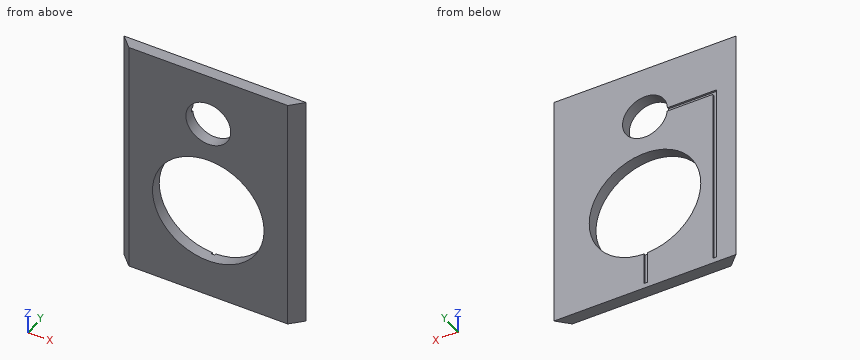
```python
from build123d import *

# Parameters (mm, degrees)
F0_W     = 300
F0_H     = 400
F1_DEPTH = 19
F2_R     = 37
F2_R_2   = 92
F3_DEPTH = 19
F4_SIZE  = 18.99999
F6_DEPTH = 3
F7_W     = 6
F7_H     = 64.6666483516
F8_DEPTH = 3


# Not quite as in the source:
# - a fillet or chamfer is up to 0.001 mm smaller than in the source, because OpenCascade refuses the exact size


with BuildPart() as f1:
    # F0 (on Front) → F1 (new body)
    with BuildSketch(Plane.XZ):
        with Locations((-100.0432893634, -3.2491389651)):
            Rectangle(F0_W, F0_H)
    extrude(amount=F1_DEPTH)

    # F2 (on face) → F3 (cut)
    with BuildSketch(Plane.XZ.offset(19)):
        with Locations((-100.0432893634, 109.7508610349)):
            Circle(F2_R)
        with Locations((-100.0432893634, -48.7491389651)):
            Circle(F2_R_2)
    extrude(amount=-F3_DEPTH, mode=Mode.SUBTRACT)

    # F4 (size 19 in the source; OpenCascade refuses exactly that, so slightly less here)
    f4_edges = [f1.edges().sort_by_distance(p)[0] for p in [
        (-250.043289, -19, -3.249139),
        (49.956711, -19, -3.249139),
    ]]
    chamfer(f4_edges, length=F4_SIZE)

    # F5 (on face) → F6 (cut)
    with BuildSketch(Plane(origin=(0, 0, 0), x_dir=(-1, 0, 0), z_dir=(0, 1, 0))):
        Polygon((136.7686212203, 111.2508610349), (136.7686212203, 105.2508610349), (212.0432893634, 105.2508610349), (212.0432893634, -194.7491389651), (218.0432893634, -194.7491389651), (218.0432893634, 111.2508610349), align=None)
    extrude(amount=-F6_DEPTH, mode=Mode.SUBTRACT)

    # F7 (on face) → F8 (cut)
    with BuildSketch(Plane(origin=(0, 0, 0), x_dir=(-1, 0, 0), z_dir=(0, 1, 0))):
        with Locations((101.5432893634, -162.4158147893)):
            Rectangle(F7_W, F7_H)
    extrude(amount=-F8_DEPTH, mode=Mode.SUBTRACT)


solid = f1.part
```
Input: part model. Units: mm. Frame: model coordinates. Coordinates: 2 decimals unless noted, no trailing zeros. Order: outer loops, then holes, each group sorted by start corner. A loop starts at its lowest first (then second) coordinate and runs counter-clockwise, first axis right, second up. Notation, with made-up numbers: (-24.75, -7) - (-11.75, -7) arc R28 cw to (-11.75, 16) - close; hole circle Ø2 at (-31, -32). An arc over 180 degrees is marked (long way). Put each result on its own line as item: value.
1. Cut plane B-B on x = -89.5. Return the cut outline in (y, z), then the cut area to 3 significant figures.
Report:
outline: (-19, -203.25) - (0, -203.25) - (0, -140.14) - (-19, -140.14) - close; (-19, 42.64) - (0, 42.64) - (0, 74.28) - (-19, 74.28) - close; (-19, 145.22) - (0, 145.22) - (0, 196.75) - (-19, 196.75) - close
area: 2,780 mm2
2. Cut plane D-D on y = -6.75. Return the cut outline in (x, z), then the cut area to 3 significant figures.
Report:
outline: (-243.29, -203.25) - (43.21, -203.25) - (43.21, 196.75) - (-243.29, 196.75) - close; hole circle Ø184 at (-100.04, -48.75); hole circle Ø74 at (-100.04, 109.75)
area: 83,700 mm2
3. Line query: line 1 along Z through (x, y) = (-90, -3.75); line 2 along Z through (x, y) = (-68, -9); line 3 along X through (y, z) = (-5.75, 143.5). Output: solid intervals per line, ascending.
Report:
line 1: z = -203.25 to -140.2, 42.7 to 74.14, 145.36 to 196.75
line 2: z = -203.25 to -134.99, 37.49 to 91.25, 128.25 to 196.75
line 3: x = -244.29 to -115.21, -84.88 to 44.21
4. Contact query for flat-ended pins moving along their axis: pin 1 Ø24.5 at (x, z) = (-174, -111.5) entering from +Y; pin 2 Ø3.5 at (y, z) = (-2, -159) entering from +X; pin 3 Ø2 at (y, z) = (-13.5, 103) entering from +X; pin 4 Ø1.8 at (x, z) = (-102.5, -179.5) entering from +Y. Output: stop coordinate, or through.
Report:
pin 1: stops at y = 0
pin 2: stops at x = 49.71
pin 3: stops at x = 37.46
pin 4: stops at y = -3
